Here's how the part is built. I have some questions about the finished solid (model axes, mm). A direction names the side the tool comes from. Round coordinates to 2 decimals unless told otherwise and drop trailing zeros. Write each loop counter-clockwise with the first axis right and the second up, starting at its lowest first coordinate (ties: lowest second). Pieces come first, ordered by that corner, then holes. Notation, with made-up numbers: M 88,35 L 128,35 A27 cw 128,69 Z; hole C -4.75,19.25 d10. An arc over 180 degrees is marked long. Write item = value, one per line. Start each with the question number.
(1) I want a section at A-A (z = -52). List the corners of the cut face in (x, y) for me, and give its area (3 significant figures).
(2) On a 3-axis mill with a long thin cutter (end or side, diameter ignored), from which of +Z, -Z, +X, -X, +Y, -Y can I reach the whole of each face in a straight line? I mean faces 1 (the flat face through (-130, -3, -7)), 2 (the flat face through (-7, -11, -25)), 3 (the flat face through (-70, -3, -55)). Say none if no direction works.
(3) If we mould it in two halves opening along X, with no side actions, what happens to faces 4 (the flat face through (-27, -11, -25)), 5 (the flat face through (-157, -9.588, -5)), 6 (the flat face through (0, -7, -35)), 7 (the flat face through (-8.5, -11.2, -47.6))? For each: released by +X, released by -X, zero draft, split by the parting line, or undercut.
(4) I want a section at B-B (z = -62). List the corners of the cut face in (x, y) for me, and give its area (3 significant figures).
(5) I need wall thicknesses on line 1 along X through (y, z) = (-3, -25); line 2 along Z through (x, y) = (-30, 2.95); line 3 along Z through (x, y) = (-160.5, -8.25). Which ranges of each line are inside material? Lowest first, please.
(6) I want a section at C-C (x = -134). List the corners of the cut face in (y, z) for me, and give its area (3 significant figures).
(7) Will these pins go through, and if not, where does the flat tip stop? pin 1 Ø6 at (y, z) = (1, -9.5) entering from -X; pin 2 Ø3.5 at (x, z) = (-110, -45) entering from -Y; pin 3 Ø4 at (x, y) = (-89, -4) entering from -Z.
(8) I want a section at D-D (z = -35). List the corners of the cut face in (x, y) for me, and give its area (3 significant figures).
Autodesk Inventor part; units mm, degrees
ref_plane "Work Plane1" through (0, -2.75, 0) normal (0, -1, 0) x (1, 0, 0)
ref_plane "Work Plane2" through (-152.5, -8.5, -20) normal (0, 0, -1) x (-1, 0, 0)
ref_plane "Work Plane3" through (-130, -9.5, -35) normal (0, 0, -1) x (-1, 0, 0)
sketch "Sketch1" plane through (0, 0, 0) normal (0, 1, 0) x (-1, 0, 0)
  line L0 (0, 0) -> (145, 0)
  line L1 (145, 0) -> (145, -70)
  line L2 (145, -70) -> (0, -70)
  line L3 (0, -70) -> (0, 0)
  line L4 (10, -25) -> (30, -25)
  line L5 (30, -25) -> (30, -45)
  line L6 (30, -45) -> (10, -45)
  line L7 (10, -45) -> (10, -25)
  circle A0 centre (10, -25) radius 1.5
  circle A1 centre (30, -45) radius 1.5
  circle A2 centre (30, -25) radius 1.5
  circle A3 centre (10, -45) radius 1.5
  line L8 (145, 0) -> (130, 0)
  line L9 (130, 0) -> (130, -70)
  line L10 (130, -70) -> (145, -70)
  line L11 (145, -70) -> (145, 0)
  line L12 (130, -15) -> (0, -15)
  line L13 (0, -15) -> (0, -55)
  line L14 (0, -55) -> (130, -55)
  line L15 (130, -55) -> (130, -15)
  line L16 (36, -15) -> (36, -55)
  point P0 (130, 0)
  point P1 (0, -15)
  dimension "d0" = 145
  dimension "d1" = 70
  dimension "d2" = 20
  dimension "d3" = 20
  dimension "d4" = 25
  dimension "d5" = 10
  dimension "d6" = 3
  dimension "d7" = 3
  dimension "d8" = 3
  dimension "d9" = 3
  dimension "d18" = 15
  dimension "d19" = 15
  dimension "d23" = 36
  dimension "d66" = 15
extrude "Extrusion1" add sketch "Sketch1" along normal blind 4 contours L0 L1 L2 L9 | L12 L16 L14 L3 | L9 L14 L16 L12 | L4 A2 L5 A1 L6 A3 L7 A0
extrude "Extrusion2" add sketch "Sketch1" against normal blind 5.5 contours L0 L1 L2 L9 | L9 L14 L16 L12
ref_plane "Work Plane1" through (0, -2.75, 0) normal (0, -1, 0) x (1, 0, 0)
mirror "Mirror1" about plane through (0, -2.75, 0) normal (0, -1, 0) of "Extrusion1"
chamfer "Chamfer1" distance 12.5 angle 45 4 edges at (0, 2, -15) (0, -7.5, -15) (0, -7.5, -55) (0, 2, -55)
ref_plane "Work Plane2" through (-152.5, -8.5, -20) normal (0, 0, -1) x (-1, 0, 0)
sketch "Sketch5" plane through (-130, -9.5, -55) normal (0, -1, 0) x (1, 0, 0)
  circle A0 centre (100, 30) radius 1.5
  line L0 (100, 33.4641) -> (103, 31.7321)
  line L1 (103, 31.7321) -> (103, 28.2679)
  line L2 (103, 28.2679) -> (100, 26.5359)
  line L3 (100, 26.5359) -> (97, 28.2679)
  line L4 (97, 28.2679) -> (97, 31.7321)
  line L5 (97, 31.7321) -> (100, 33.4641)
  circle A1 centre (120, 30) radius 1.5
  line L6 (120, 33.4641) -> (123, 31.7321)
  line L7 (123, 31.7321) -> (123, 28.2679)
  line L8 (123, 28.2679) -> (120, 26.5359)
  line L9 (120, 26.5359) -> (117, 28.2679)
  line L10 (117, 28.2679) -> (117, 31.7321)
  line L11 (117, 31.7321) -> (120, 33.4641)
  circle A2 centre (120, 10) radius 1.5
  line L12 (120, 13.4641) -> (123, 11.7321)
  line L13 (123, 11.7321) -> (123, 8.2679)
  line L14 (123, 8.2679) -> (120, 6.5359)
  line L15 (120, 6.5359) -> (117, 8.2679)
  line L16 (117, 8.2679) -> (117, 11.7321)
  line L17 (117, 11.7321) -> (120, 13.4641)
  circle A3 centre (100, 10) radius 1.5
  line L18 (100, 13.4641) -> (103, 11.7321)
  line L19 (103, 11.7321) -> (103, 8.2679)
  line L20 (103, 8.2679) -> (100, 6.5359)
  line L21 (100, 6.5359) -> (97, 8.2679)
  line L22 (97, 8.2679) -> (97, 11.7321)
  line L23 (97, 11.7321) -> (100, 13.4641)
  circle A4 centre (100, 30) radius 5.25
  circle A5 centre (120, 30) radius 5.25
  circle A6 centre (120, 10) radius 5.25
  circle A7 centre (100, 10) radius 5.25
  point P0 (130, 55)
  dimension "d44" = 6
  dimension "d45" = 6
  dimension "d46" = 6
  dimension "d47" = 6
  dimension "d48" = 10.5
  dimension "d49" = 10.5
  dimension "d50" = 10.5
  dimension "d51" = 10.5
extrude "Extrusion5" add sketch "Sketch5" along normal blind 3.5 contours A4 | A5 | A6 | A7
sketch "Sketch6" plane through (-130, -9.5, -55) normal (0, -1, 0) x (1, 0, 0)
  circle A0 centre (0, 10) radius 1.5
  line L0 (117.5, 0) -> (0, 0)
  line L1 (0, 0) -> (0, -15)
  circle A1 centre (20, 10) radius 1.5
  circle A2 centre (40, 10) radius 1.5
  circle A3 centre (60, 10) radius 1.5
  point P0 (130, 55)
  point P1 (0, -5)
  dimension "d54" = 3
  dimension "d55" = 10
  dimension "d56" = 0
  dimension "d59" = 20
extrude "Extrusion6" cut sketch "Sketch6" against normal blind 33.25
ref_plane "Work Plane3" through (-130, -9.5, -35) normal (0, 0, -1) x (-1, 0, 0)
mirror "Mirror2" about plane through (-130, -9.5, -35) normal (0, 0, -1) of "Extrusion6"
sketch "Sketch7" plane through (-145, 4, 0) normal (0, 0, 1) x (1, 0, 0)
  point P0 (145, -4)
sketch "Sketch8" plane through (-145, 4, 0) normal (0, 0, 1) x (1, 0, 0)
  line L0 (0, 0) -> (15, 0)
  line L1 (15, 0) -> (0, 0)
  circle A0 centre (-25, -6.7937) radius 1.5
  circle A1 centre (-25, -6.7937) radius 7
  line L2 (0, -13.5) -> (0, 0)
  line L3 (0, -13.5) -> (0, 0)
  line L4 (-50, -13.5875) -> (0, -13.5875)
  line L5 (0, -13.5875) -> (0, 0)
  line L6 (0, 0) -> (-50, 0)
  line L7 (-50, 0) -> (-50, -13.5875)
  line L8 (-50, -13.5875) -> (0, 0) construction
  line L9 (0, -13.5875) -> (-50, 0) construction
  point P0 (145, -4)
  point P1 (-10, -1.851)
  point P2 (-10, -11.649)
  point P3 (-26.6868, -13.5875)
  point P4 (-26.6868, 0)
  point P5 (-23.3132, 0)
  point P6 (-23.3132, -13.5875)
  dimension "d72" = 3
  dimension "d73" = 14
  dimension "d74" = 25
extrude "Extrusion7" add sketch "Sketch8" against normal blind 10 contours A1 L4 L6 | A1 L6 L2 L5 L4 | L6 A1 | A1 L4
ref_plane "Work Plane4" through (-130, -9.5, -35) normal (0, 0, 1) x (1, 0, 0)
mirror "Mirror3" about plane through (-130, -9.5, -35) normal (0, 0, 1) of "Extrusion7"
properties part number "RobotBaseMotorExt"
Returned:
q1.outline = M -145,-9.5 L -9.5,-9.5 L -9.5,-5.5 L -36,-5.5 L -36,0 L -9.5,0 L -9.5,4 L -145,4 Z
q1.area = 1,680 mm²
q2.face_1 = +Z, +X, +Y, -Y
q2.face_2 = -Y
q2.face_3 = -Z, +X, +Y, -Y
q3.face_4 = undercut
q3.face_5 = zero draft
q3.face_6 = released by +X
q3.face_7 = undercut
q4.outline = M -168.31,-9.59 L -145,-9.59 L -145,-9.5 L -130,-9.5 L -130,4 L -168.31,4 A7 ccw long Z; hole C -170,-2.79 d3
q4.area = 613 mm²
q5.line_1 = -145 to -131.5, -128.5 to -111.5, -108.5 to -91.5, -88.5 to -71.5, -68.5 to -36
q5.line_2 = -55 to -46.5, -43.5 to -26.5, -23.5 to -15
q5.line_3 = -70 to -60, -10 to 0
q6.outline = M -9.5,-70 L 4,-70 L 4,0 L -9.5,0 Z
q6.area = 945 mm²
q7.pin_1 = -176.95
q7.pin_2 = -9.5
q7.pin_3 = -55
q8.outline = M -145,-9.5 L 0,-9.5 L 0,-5.5 L -36,-5.5 L -36,0 L 0,0 L 0,4 L -145,4 Z
q8.area = 1,760 mm²
